```python
from build123d import *

# Parameters (mm, degrees)
F0_W     = 17
F0_H     = 11.425
F0_R     = 2.5
F1_DEPTH = 4
F3_DEPTH = 2
F4_R     = 1.7
F5_DEPTH = 11.426


with BuildPart() as f1:
    # F0 (on Top) → F1 (new body)
    with BuildSketch(Plane.XY):
        with Locations((-34.827103, 23.066922)):
            Rectangle(F0_W, F0_H)
        with Locations((-34.827103, 24.279422)):
            Circle(F0_R, mode=Mode.SUBTRACT)
    extrude(amount=F1_DEPTH)

    # F2 (on face) → F3 (join)
    with BuildSketch(Plane(origin=(0, 0, 0), x_dir=(1, 0, 0), z_dir=(0, 0, -1))):
        with BuildLine():
            ThreePointArc((-38.577103, -24.279422), (-34.827103, -20.529422), (-31.077103, -24.279422))
            Line((-31.077103, -24.279422), (-31.077103, -28.779422))
            Line((-31.077103, -28.779422), (-26.327103, -28.779422))
            Line((-26.327103, -28.779422), (-26.327103, -17.354422))
            Line((-26.327103, -17.354422), (-43.327103, -17.354422))
            Line((-43.327103, -17.354422), (-43.327103, -28.779422))
            Line((-43.327103, -28.779422), (-38.577103, -28.779422))
            Line((-38.577103, -28.779422), (-38.577103, -24.279422))
        make_face()
    extrude(amount=F3_DEPTH)

    # F4 (on face) → F5 (cut, through all)
    with BuildSketch(Plane.XZ.offset(-17.354422)):
        with Locations((-28.827103, 1)):
            Circle(F4_R)
        with Locations((-40.827103, 1)):
            Circle(F4_R)
    extrude(amount=-F5_DEPTH, mode=Mode.SUBTRACT)


solid = f1.part
```
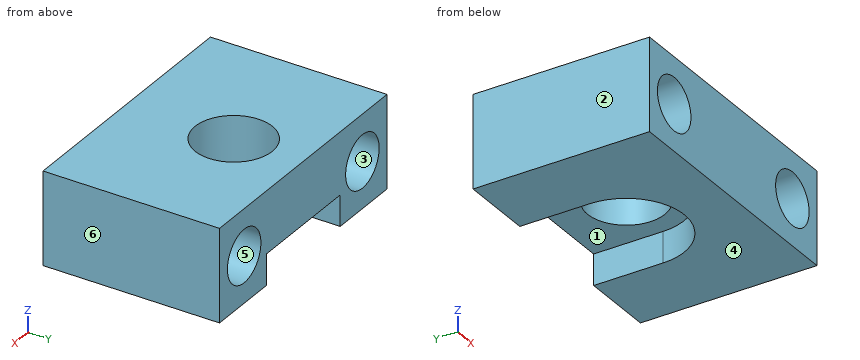
Source: CAD feature listing. Evaluate the final solid. Frame: model axes, mm. Face numbers are marked on the shaded views. A direction names the side the tool comes from. Give positions to 0.01 mm unless a question says otherwise; leave off trailing zeros. Loops run counter-clockwise (first coordinate to the right, second up) from the corner with the lowest first, then second, coordinate; pieces in that order, holes last. Notation, with made-up numbers: (21, 1.25) - (41, 1.25) arc R30 ccw to (41, 32.25) - close; hole circle Ø6 at (-37.75, -23.75). An arc over 180 degrees is marked (long way). Use CSV: the item, a comma, the result in double quotes. Start each with the question number.
1. Ray query, L1, parallel to X at y = 26.75, z = -0.15; L2, parallel to X at y = 25.5, z = 0.35; L3, parallel to Z at x = -36.5, y = 21.25. Return the intervals inside material, ascending.
2. Section D-D (y = 28.25). Output: boundary loops of the cut face in (x, z).
3. Section B-B (y = 22). Output: boundary loops of the cut face in (x, z).
4. Reachability of the marked faces 1 and 2 from +Z, -Z, +X, -X, +Y, -Y: full face, straight path, thin tool, end or side. Return the list, or none.
5. Section C-C (x = -29.5). Output: boundary loops of the cut face in (y, z).
6. Section A-A (z = 1). Output: boundary loops of the cut face in (x, y).
7. Draft query along Z for the marked faces 3, 4, 5 and 6. Return one class per face: +Z half, -Z half, draft (parallel to the pull), parting line (faces both ways), or undercut.
Response:
1,L1,"-43.33 to -42.08, -39.58 to -38.58, -31.08 to -30.08, -27.58 to -26.33"
1,L2,"-43.33 to -42.4, -39.26 to -37.01, -32.65 to -30.4, -27.26 to -26.33"
1,L3,"0 to 4"
2,outline,"(-43.33, -2) - (-38.58, -2) - (-38.58, 0) - (-31.08, 0) - (-31.08, -2) - (-26.33, -2) - (-26.33, 4) - (-43.33, 4) - close; hole circle Ø3.4 at (-40.83, 1); hole circle Ø3.4 at (-28.83, 1)"
3,outline,"(-43.33, -2) - (-37.8, -2) - (-37.8, 0) - (-35.85, 0) - (-35.85, 4) - (-43.33, 4) - close; (-33.8, 0) - (-31.85, 0) - (-31.85, -2) - (-26.33, -2) - (-26.33, 4) - (-33.8, 4) - close; hole circle Ø3.4 at (-40.83, 1); hole circle Ø3.4 at (-28.83, 1)"
4,face 1,"-Z, +Y"
4,face 2,"+Z, -Z, -X, +Y, -Y"
5,outline,"(17.35, -2) - (28.78, -2) - (28.78, -0.56) - (17.35, -0.56) - close; (17.35, 2.56) - (28.78, 2.56) - (28.78, 4) - (17.35, 4) - close"
6,outline,"(-43.33, 17.35) - (-42.53, 17.35) - (-42.53, 28.78) - (-43.33, 28.78) - close; (-39.13, 17.35) - (-30.53, 17.35) - (-30.53, 28.78) - (-39.13, 28.78) - close; (-27.13, 17.35) - (-26.33, 17.35) - (-26.33, 28.78) - (-27.13, 28.78) - close; hole circle Ø5 at (-34.83, 24.28)"
7,face 3,"undercut"
7,face 4,"-Z half"
7,face 5,"undercut"
7,face 6,"draft"
